```python
from build123d import *

# Parameters (mm, degrees)
SALIENTE_EXTRUIR1_DEPTH = 24
CORTAR_EXTRUIR1_DEPTH   = 1


with BuildPart() as part:
    # Croquis1 → Saliente-Extruir1 (new body)
    with BuildSketch(Plane.XY):
        with BuildLine():
            Line((0, 3), (-70, 3))
            Line((-70, 3), (-70, 2.5))
            Line((-70, 2.5), (0, 2.5))
            ThreePointArc((0, 2.5), (0.835770646, -2.356159466), (-1.575367134, 1.941189942))
            Line((-1.575367134, 1.941189942), (-1.890440561, 2.329427931))
            ThreePointArc((-1.890440561, 2.329427931), (1.002924775, -2.827391359), (0, 3))
        make_face()
    extrude(amount=SALIENTE_EXTRUIR1_DEPTH)

    # Croquis2 → Cortar-Extruir1 (cut)
    with BuildSketch(Plane(origin=(0, 3, 0), x_dir=(1, 0, 0), z_dir=(0, 1, 0))):
        with BuildLine():
            Line((-58, -10.5), (-33, -10.5))
            ThreePointArc((-33, -10.5), (-31.5, -12), (-33, -13.5))
            Line((-33, -13.5), (-58, -13.5))
            ThreePointArc((-58, -13.5), (-59.5, -12), (-58, -10.5))
        make_face()
        with BuildLine():
            Line((-58, 0), (-75.765424477, 0))
            Line((-75.765424477, 0), (-75.765424477, -24))
            Line((-75.765424477, -24), (-58, -24))
            ThreePointArc((-58, -24), (-70, -12), (-58, 0))
        make_face()
    extrude(amount=-CORTAR_EXTRUIR1_DEPTH, mode=Mode.SUBTRACT)


solid = part.part
```
Geometry: final body of the model. Coordinates: model frame, mm. Coordinates: 2 decimals unless noted, no trailing zeros. Order: outer loops, then holes, each group sorted by start corner. A loop starts at its lowest first (then second) coordinate and runs counter-clockwise, first axis right, second up. Notation, with made-up numbers: (3, -25.75) - (9, -25.75) arc R25 ccw to (9, 4.25) - close; hole circle Ø2 at (24, -15.5). An arc over 180 degrees is marked (long way). Return JSON: item names as keys, results as strings. Group by question number.
1. Cut plane C-C (y = 0). Output: boundary loops of the cut face in (x, z), plus the area to 3 significant figures.
2. Pin query (flat end, axial travel): pin 1 (6 mm diameter, centred on x = -8, z = 14, fed in from -Y); pin 2 (2 mm diameter, centred on y = 1.5, z = 15, fed in from +X). Return the tip coordinate at first contact, or that it passes through.
3. Material intervals for line 1 along X through (y, z) = (-0.25, 3); line 2 along Y through (x, z) = (-41.5, 18); line 3 along X through (y, z) = (-2.25, 10.75), sorted ascending. Write a range as [from, to].
4. Pull-direction query (X, two-part tool) for faces 1 (the face through (0.891, -2.865, 11.832)), 2 (the face through (-31.5, 2.8, 12)), 3 (the face through (-59.5, 2.8, 12)), 4 (the face through (-35, 3, 9)); classes: pulls with the +X half, pulls with the -X half, needs draft (parallel to the pull), parting line crosses it, or undercut.
5. Cut plane D-D (x = -10.5). Output: boundary loops of the cut face in (y, z).
6. Cut plane B-B (x = -35). Output: boundary loops of the cut face in (y, z).
7. Cut plane A-A (z = 12). Output: boundary loops of the cut face in (x, y), plus the area to 3 significant figures.
Resolved:
{
 "1": {"outline": "(-3, 0) - (-2.5, 0) - (-2.5, 24) - (-3, 24) - close; (2.5, 0) - (3, 0) - (3, 24) - (2.5, 24) - close", "area": "24.0 mm²"},
 "2": {"pin 1": "stops at y = 2.5", "pin 2": "stops at x = 2.96"},
 "3": {"line 1": "x = [-2.99, -2.49], [2.49, 2.99]", "line 2": "y = [2.5, 3]", "line 3": "x = [-1.98, -1.09], [1.09, 1.98]"},
 "4": {"face 1": "parting line crosses it", "face 2": "undercut", "face 3": "undercut", "face 4": "needs draft"},
 "5": {"outline": "(2.5, 0) - (3, 0) - (3, 24) - (2.5, 24) - close"},
 "6": {"outline": "(2.5, 0) - (3, 0) - (3, 10.5) - (2.5, 10.5) - close; (2.5, 13.5) - (3, 13.5) - (3, 24) - (2.5, 24) - close"},
 "7": {"outline": "(-70, 2.5) - (-59.5, 2.5) - (-59.5, 3) - (-70, 3) - close; (-31.5, 2.5) - (0, 2.5) arc R2.5 cw (long way) to (-1.58, 1.94) - (-1.89, 2.33) arc R3 ccw (long way) to (0, 3) - (-31.5, 3) - close", "area": "28.7 mm²"}
}
